```python
from build123d import *

# Parameters (mm, degrees)
BOSS_EXTRUDE1_DEPTH     = 20
SKETCH2_R               = 12.7
BOSS_EXTRUDE2_DEPTH     = 30
FILLET1_R               = 20
CUT_EXTRUDE1_DEPTH      = 111.630296483
CUT_EXTRUDE1_DEPTH_BACK = 111.630296483
SKETCH3_R               = 12.7


with BuildPart() as part:
    # Sketch1 → Boss-Extrude1 (new, symmetric)
    with BuildSketch(Plane.XY):
        with BuildLine():
            Line((-40, 70), (-40, 0))
            Line((-40, 0), (40, 0))
            Line((40, 0), (40, 70))
            ThreePointArc((40, 70), (36.25, 73.75), (32.5, 70))
            Line((32.5, 70), (32.5, 7.5))
            Line((32.5, 7.5), (-32.5, 7.5))
            Line((-32.5, 7.5), (-32.5, 70))
            ThreePointArc((-32.5, 70), (-36.25, 73.75), (-40, 70))
        make_face()
    extrude(amount=BOSS_EXTRUDE1_DEPTH, both=True)

    # Sketch2 → Boss-Extrude2 (add)
    with BuildSketch(Plane(origin=(0, 0, 0), x_dir=(-1, 0, 0), z_dir=(0, -1, 0))):
        with Locations(Location((0, 0, 0), (0, 0, 180))):
            Circle(SKETCH2_R)
    extrude(amount=BOSS_EXTRUDE2_DEPTH)

    # Fillet1
    fillet1_edges = [part.edges().sort_by_distance(p)[0] for p in [
        (-32.5, 7.5, 0),
        (32.5, 7.5, 0),
        (40, 0, 0),
        (-40, 0, 0),
    ]]
    fillet(fillet1_edges, radius=FILLET1_R)

    # Sketch3 → Cut-Extrude1 (cut, two sides: drawn at the far end of the back side and taken through both)
    with BuildSketch(Plane.ZY.offset(40).offset(-CUT_EXTRUDE1_DEPTH_BACK)):
        with Locations((0, 54)):
            Circle(SKETCH3_R)
    extrude(amount=CUT_EXTRUDE1_DEPTH + CUT_EXTRUDE1_DEPTH_BACK, mode=Mode.SUBTRACT)


solid = part.part
```
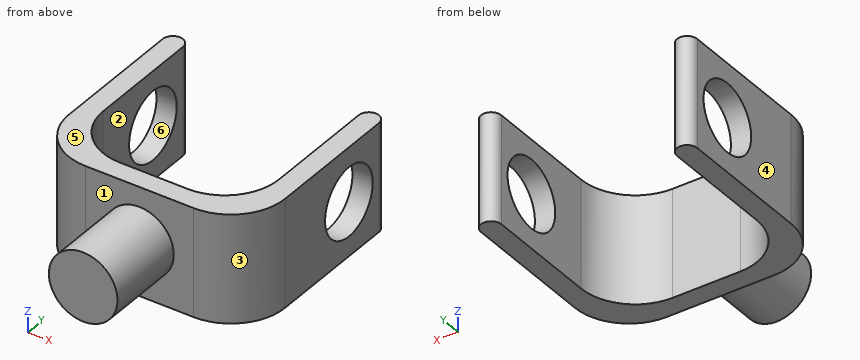
CAD build for the part. Positions are in the model's coordinates, mm. Face numbers are marked on the shaded views. A direction names the side the tool comes from. Round coordinates to 2 decimals unless told otherwise and drop trailing zeros. Write each loop counter-clockwise with the first axis right and the second up, starting at its lowest first coordinate (ties: lowest second). Pieces come first, ordered by that corner, then holes. Notation, with made-up numbers: M 52,12 L 59,12 A28 cw 59,37 Z; hole C -39,72.25 d8. An arc over 180 degrees is marked long. One line per question, with ' | ' between items.
1. Cut at C-C on y = 54. Write the cut outline in (x, z).
Working result:
outline: M -40,-20 L -32.5,-20 L -32.5,-12.7 L -40,-12.7 Z; M -40,12.7 L -32.5,12.7 L -32.5,20 L -40,20 Z; M 32.5,-20 L 40,-20 L 40,-12.7 L 32.5,-12.7 Z; M 32.5,12.7 L 40,12.7 L 40,20 L 32.5,20 Z
2. Mould opens along Z. For the marked faces 4, 5 and 6 say: pulls with the +Z half, pulls with the -Z half, needs draft (parallel to the pull), parting line crosses it, or undercut.
Working result:
face 4: needs draft | face 5: pulls with the +Z half | face 6: undercut
3. Probe L1, parallel to Z at x = 35.5, y = 54; L2, parallel to X at y = 19, z = -8; L3, parallel to Y at x = -37, z = 0. List the from-to ranges inside material, lowest first. Write a range as from..to.
Working result:
L1: -20..-12.7, 12.7..20 | L2: -39.97..-30.6, 30.6..39.97 | L3: 9.46..41.3, 66.7..73.67
4. Pin check, flat tips, straight feed: pin 1 Ø1.5 at (y, z) = (-1.5, 4.5) entering from +X; pin 2 Ø2 at (x, y) = (-31, 46) entering from +Z; pin 3 Ø8 at (x, z) = (-18, -7.5) entering from +Y; pin 4 Ø1 at (y, z) = (12.5, -9.5) entering from +X (3 decimals). Stop position of each tip, or through.
Working result:
pin 1: x = 12.13 | pin 2: through | pin 3: y = 9.9 | pin 4: x = 38.735
5. Cut at D-D on z = -15. Write the cut outline in (x, y).
Working result:
outline: M -40,20 A20 ccw -20,0 L 20,0 A20 ccw 40,20 L 40,70 A3.75 ccw 32.5,70 L 32.5,27.5 A20 cw 12.5,7.5 L -12.5,7.5 A20 cw -32.5,27.5 L -32.5,70 A3.75 ccw -40,70 Z
6. Cut at A-A on z = 0. Write the cut outline in (x, y).
Working result:
outline: M -40,20 A20 ccw -20,0 L -12.7,0 L -12.7,-30 L 12.7,-30 L 12.7,0 L 20,0 A20 ccw 40,20 L 40,41.3 L 32.5,41.3 L 32.5,27.5 A20 cw 12.5,7.5 L -12.5,7.5 A20 cw -32.5,27.5 L -32.5,41.3 L -40,41.3 Z; M -40,66.7 L -32.5,66.7 L -32.5,70 A3.75 ccw -40,70 Z; M 32.5,66.7 L 40,66.7 L 40,70 A3.75 ccw 32.5,70 Z
7. Cut at B-B on y = 36.5. Write the cut outline in (x, z), and give its area (3 significant figures).
Working result:
outline: M -40,-20 L -32.5,-20 L -32.5,20 L -40,20 Z; M 32.5,-20 L 40,-20 L 40,20 L 32.5,20 Z | area: 600 mm2
8. Which spindle directions (+Z, -Z, +X, -X, +Y, -Y) get a long thin tool onto all of the face, cutting with end or side? Do the marked faces 1, 2 and 3. Say none if no direction does.
Working result:
face 1: -Y | face 2: +Z, -Z, +Y | face 3: +Z, -Z, +X, -Y
